from build123d import *

# Parameters (mm, degrees)
SKETCH1_R           = 50
BOSS_EXTRUDE1_DEPTH = 20
SKETCH2_R           = 67.8
SKETCH2_R_2         = 50
CUT_EXTRUDE2_DEPTH  = 10


with BuildPart() as part:
    # Sketch1 → Boss-Extrude1 (new body)
    with BuildSketch(Plane(origin=(0, 0, 0), x_dir=(1, 0, 0), z_dir=(0, 1, 0))):
        with BuildLine():
            Line((172.912878475, 10), (188.729833462, 10))
            ThreePointArc((188.729833462, 10), (171.097880047, 33.983517439), (141.78172432, 39.146646662))
            ThreePointArc((141.78172432, 39.146646662), (87.249696592, 45.62224876), (36.143045028, 65.716666806))
            ThreePointArc((36.143045028, 65.716666806), (0, 75), (-36.143045028, 65.716666806))
            ThreePointArc((-36.143045028, 65.716666806), (-90.451837404, 44.84292871), (-148.370630479, 39.313798563))
            ThreePointArc((-148.370630479, 39.313798563), (-173.844765312, 31.461724235), (-188.728411831, 9.346939972))
            Line((-188.728411831, 9.346939972), (-172.911456843, 9.346939972))
            ThreePointArc((-172.911456843, 9.346939972), (-124.998578369, -0.653060028), (-172.911456843, -10.653060028))
            Line((-172.911456843, -10.653060028), (-188.728411831, -10.653060028))
            ThreePointArc((-188.728411831, -10.653060028), (-173.704720096, -32.871359866), (-148.022685389, -40.604228308))
            ThreePointArc((-148.022685389, -40.604228308), (-90.057943753, -45.628827643), (-35.569454559, -66.028886878))
            ThreePointArc((-35.569454559, -66.028886878), (0.322743626, -74.999305574), (36.136409347, -65.720315881))
            ThreePointArc((36.136409347, -65.720315881), (90.458572132, -44.849413277), (148.389781211, -39.3297249))
            ThreePointArc((148.389781211, -39.3297249), (173.396792242, -31.654544351), (188.071249852, -10))
            Line((188.071249852, -10), (172.912878475, -10))
            ThreePointArc((172.912878475, -10), (125, 0), (172.912878475, 10))
        make_face()
        with Locations(Location((0, 0, 0), (0, 0, 270))):
            Circle(SKETCH1_R, mode=Mode.SUBTRACT)
    extrude(amount=BOSS_EXTRUDE1_DEPTH)

    # Sketch2 → Cut-Extrude2 (cut)
    with BuildSketch(Plane(origin=(0, 0, 0), x_dir=(1, 0, 0), z_dir=(0, 1, 0))):
        with Locations(Location((0, 0, 0), (0, 0, 270))):
            Circle(SKETCH2_R)
        with Locations(Location((0, 0, 0), (0, 0, 270))):
            Circle(SKETCH2_R_2, mode=Mode.SUBTRACT)
    extrude(amount=CUT_EXTRUDE2_DEPTH, mode=Mode.SUBTRACT)


solid = part.part
Design review of the part built by this model. Coordinates are the model's own, in mm. A direction names the side the tool comes from. Round coordinates to 2 decimals unless told otherwise and drop trailing zeros. Write each loop counter-clockwise with the first axis right and the second up, starting at its lowest first coordinate (ties: lowest second). Pieces come first, ordered by that corner, then holes.
Item 1: For faces 4 (the flat face through (-181, 10, -9.347)), 5 (the cylindrical face through (67.223, 4.93, -8.826)), 6 (the flat face through (181, 10, 10)), list the 3-axis set-ups (+Z, -Z, +X, -X, +Y, -Y) from which the entire face can be reached by the end or side of a thin tool; tool diameter is ignored.
Item 2: Consider section A-A on x = 0. Give the boundary of the cut face in (y, z), and give its area (3 significant figures).
Item 3: Wall thickness on L1, parallel to X at y = 15, z = 0; L2, parallel to X at y = 7.5, z = 0; L3, parallel to Z at x = 150, y = 4.75: over which ranges is each line inside the solid? List them lowest first.
Item 4: Consider section C-C on y = 4.75. Give the boundary of the cut face in (x, z).
Item 5: Consider section D-D on z = 58. Give the boundary of the cut face in (x, y), and give its area (3 significant figures).
Item 6: Consider section B-B on z = 31.5. Give the boundary of the cut face in (x, y).
Item 7: For pin 1 Ø4.5 at (x, y) = (-181.5, 6.5) entering from +Z; pin 2 Ø10 at (x, y) = (-10.5, 3) entering from +Z; pin 3 Ø6 at (x, y) = (127, 12.5) entering from +Z, all flat-tipped, find the tip position at first contact; note any pin that passes through.
Item 8: Draft analysis for pull direction X (two halves, no side actions). For faces 1 (the cylindrical face through (87.998, 9.86, -45.436)), 2 (the cylindrical face through (0, 10, 75)), 3 (the flat face through (-181, 10, 10.653)), state which applies: released by +X, released by -X, zero draft, split by the parting line, or undercut.
Check values:
1. face 4: -X, +Y, -Y
1. face 5: -Y
1. face 6: +X, +Y, -Y
2. outline: (0, -75) - (20, -75) - (20, -50) - (10, -50) - (10, -67.8) - (0, -67.8) - close; (0, 67.8) - (10, 67.8) - (10, 50) - (20, 50) - (20, 75) - (0, 75) - close
2. area: 644 mm2
3. L1: x = -125.01 to -50, 50 to 125
3. L2: x = -125.01 to -67.8, 67.8 to 125
3. L3: z = -40 to -25, 25 to 39.36
4. outline: (-188.73, -9.35) arc R40 ccw to (-148.37, -39.31) arc R214.75 cw to (-36.14, -65.72) arc R75 ccw to (36.14, -65.72) arc R214.75 cw to (141.78, -39.15) arc R40 ccw to (188.73, -10) - (172.91, -10) arc R25 cw (long way) to (172.91, 10) - (188.07, 10) arc R39.36 ccw to (148.39, 39.33) arc R214.75 cw to (36.14, 65.72) arc R75 ccw to (-35.57, 66.03) arc R214.75 cw to (-148.02, 40.6) arc R40 ccw to (-188.73, 10.65) - (-172.91, 10.65) arc R25 cw (long way) to (-172.91, -9.35) - close; hole circle Ø135.6 at (0, 0)
5. outline: (-52.14, 0) - (-35.11, 0) - (-35.11, 10) - (35.11, 10) - (35.11, 0) - (51.62, 0) - (51.62, 20) - (-52.14, 20) - close
5. area: 1,370 mm2
6. outline: (-175.46, 0) - (-60.04, 0) - (-60.04, 10) - (-38.83, 10) - (-38.83, 20) - (-175.46, 20) - close; (38.83, 10) - (60.04, 10) - (60.04, 0) - (173.6, 0) - (173.6, 20) - (38.83, 20) - close
7. pin 1: stops at z = 27.94
7. pin 2: stops at z = 74.8
7. pin 3: stops at z = 39.72
8. face 1: undercut
8. face 2: split by the parting line
8. face 3: zero draft
